Can you work these out from the model? Positions are in its coordinate system, mm. Give positions to 0.01 mm unless a question says otherwise; leave off trailing zeros. Order: outer loops, then holes, each group sorted by start corner. A loop starts at its lowest first (then second) coordinate and runs counter-clockwise, first axis right, second up. Notation, with made-up numbers: M -30,44 L 14,44 A23 ccw 14,67 Z; hole C -7.75,-24.5 d6. An arc over 180 degrees is marked long. Use one line per item in the form item = value. Start each with the question number.
1. I need wall thicknesses on L1, parallel to X at y = -0.3, z = -3; L2, parallel to Z at x = 36, y = 0.2; L3, parallel to X at y = 0.8, z = 2.5. Which ranges of each line are inside material? Lowest first, please.
2. I want a section at B-B, the plane y = 1.1. Count the separate pieces of the cut face and the enclosed holes in it, and give its area (3 significant figures).
3. Will these pins go through, and if not, where does the flat tip stop? P1, Ø0.5, axis at y = 1, z = -7, coming from the +X side; P2, Ø0.5, axis at y = 0.5, z = 9.5, coming from the -X side.
4. I want a section at A-A, the plane x = 13.5. List the corners of the cut face in (y, z) for me (3 decimals).
5. I want a section at C-C, the plane z = -5.5. List the corners of the cut face in (x, y) for me (3 decimals).
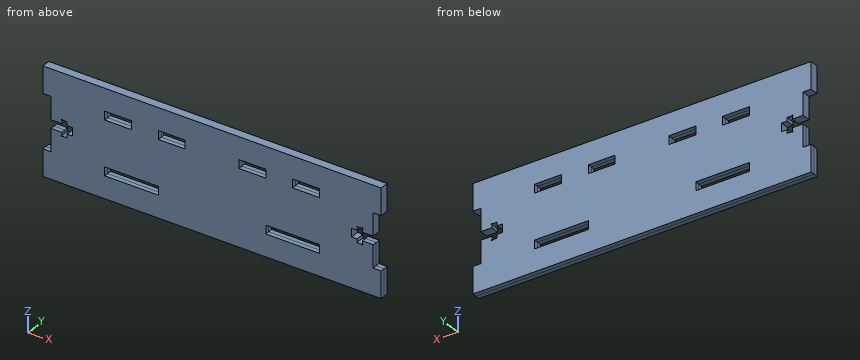
```python
from build123d import *

# Parameters (mm, degrees)
F0_W     = 20
F0_H     = 3.2
F0_W_2   = 10
F1_DEPTH = 1.585


with BuildPart() as f1:
    # F0 (on Front) → F1 (new body, symmetric)
    with BuildSketch(Plane.XZ):
        with BuildLine():
            Line((63, 20), (0, 20))
            Line((0, 20), (-63, 20))
            Line((-63, 20), (-63, 10))
            Line((-63, 10), (-60, 10))
            Line((-60, 10), (-60, 1.55))
            Line((-60, 1.55), (-56, 1.55))
            Line((-56, 1.55), (-56, 2.65))
            ThreePointArc((-56, 2.65), (-56.1767766953, 3.0767766953), (-55.75, 2.9))
            Line((-55.75, 2.9), (-54, 2.9))
            Line((-54, 2.9), (-54, 1.55))
            Line((-54, 1.55), (-52, 1.55))
            Line((-52, 1.55), (-52, 0))
            Line((-52, 0), (-52, -1.55))
            Line((-52, -1.55), (-54, -1.55))
            Line((-54, -1.55), (-54, -2.9))
            Line((-54, -2.9), (-55.75, -2.9))
            ThreePointArc((-55.75, -2.9), (-56.1767766953, -3.0767766953), (-56, -2.65))
            Line((-56, -2.65), (-56, -1.55))
            Line((-56, -1.55), (-60, -1.55))
            Line((-60, -1.55), (-60, -10))
            Line((-60, -10), (-63, -10))
            Line((-63, -10), (-63, -20))
            Line((-63, -20), (0, -20))
            Line((0, -20), (63, -20))
            Line((63, -20), (63, -10))
            Line((63, -10), (60, -10))
            Line((60, -10), (60, -1.55))
            Line((60, -1.55), (56, -1.55))
            Line((56, -1.55), (56, -2.65))
            ThreePointArc((56, -2.65), (56.1767766953, -2.7232233047), (56.25, -2.9))
            ThreePointArc((56.25, -2.9), (56, -3.15), (55.75, -2.9))
            Line((55.75, -2.9), (54, -2.9))
            Line((54, -2.9), (54, -1.55))
            Line((54, -1.55), (52, -1.55))
            Line((52, -1.55), (52, 0))
            Line((52, 0), (52, 1.55))
            Line((52, 1.55), (54, 1.55))
            Line((54, 1.55), (54, 2.9))
            Line((54, 2.9), (55.75, 2.9))
            ThreePointArc((55.75, 2.9), (56, 3.15), (56.25, 2.9))
            ThreePointArc((56.25, 2.9), (56.1767766953, 2.7232233047), (56, 2.65))
            Line((56, 2.65), (56, 1.55))
            Line((56, 1.55), (60, 1.55))
            Line((60, 1.55), (60, 10))
            Line((60, 10), (63, 10))
            Line((63, 10), (63, 20))
        make_face()
        with Locations((-30, -10.1)):
            Rectangle(F0_W, F0_H, mode=Mode.SUBTRACT)
        with Locations((30, -10.1)):
            Rectangle(F0_W, F0_H, mode=Mode.SUBTRACT)
        with Locations((-35, 10.1)):
            Rectangle(F0_W_2, F0_H, mode=Mode.SUBTRACT)
        with Locations((-15, 10.1)):
            Rectangle(F0_W_2, F0_H, mode=Mode.SUBTRACT)
        with Locations((15, 10.1)):
            Rectangle(F0_W_2, F0_H, mode=Mode.SUBTRACT)
        with Locations((35, 10.1)):
            Rectangle(F0_W_2, F0_H, mode=Mode.SUBTRACT)
    extrude(amount=F1_DEPTH, both=True)


solid = f1.part
```
Check result:
q1.L1 = -60 to -56.23, -55.77 to 55.77, 56.23 to 60
q1.L2 = -20 to -11.7, -8.5 to 8.5, 11.7 to 20
q1.L3 = -60 to -56, -54 to 54, 56 to 60
q2.separate_pieces = 1
q2.enclosed_holes = 6
q2.area = 4,600 mm2
q3.P1 = 60
q3.P2 = -60
q4.outline = M -1.585,-20 L 1.585,-20 L 1.585,8.5 L -1.585,8.5 Z; M -1.585,11.7 L 1.585,11.7 L 1.585,20 L -1.585,20 Z
q5.outline = M -60,-1.585 L 60,-1.585 L 60,1.585 L -60,1.585 Z
